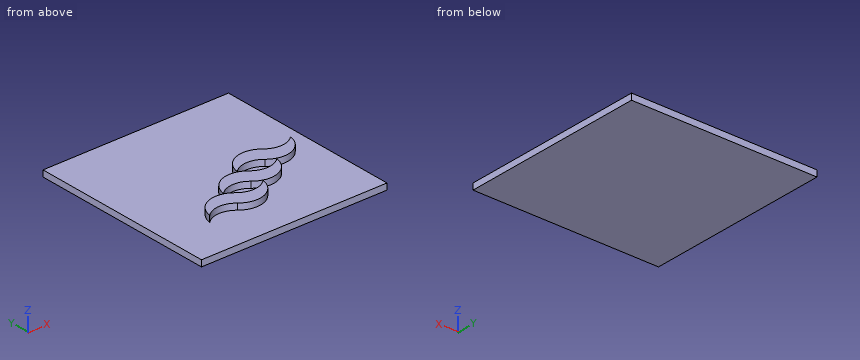
```python
from build123d import *

# Parameters (mm, degrees)
SKICA1_W                = 300
SKICA1_H                = 300
P_IDAT_VYSUNUT_M1_DEPTH = 10
P_IDAT_VYSUNUT_M3_DEPTH = 10


with BuildPart() as part:
    # Skica1 → Přidat vysunutím1 (new body)
    with BuildSketch(Plane.XY):
        with Locations((150, 150)):
            Rectangle(SKICA1_W, SKICA1_H)
    extrude(amount=P_IDAT_VYSUNUT_M1_DEPTH)

    # Skica3 → Přidat vysunutím3 (add)
    with BuildSketch(Plane.XY.offset(10)):
        with BuildLine():
            ThreePointArc((115.351436594, 67.036617417), (152.787337691, 60.386270146), (176.568555926, 90.053212507))
            ThreePointArc((176.568555926, 90.053212507), (153.853792867, 80.346404756), (130.562326016, 88.573807107))
            ThreePointArc((130.562326016, 88.573807107), (93.126424919, 95.224154378), (69.345206683, 65.557212017))
            ThreePointArc((69.345206683, 65.557212017), (92.059969742, 75.264019769), (115.351436594, 67.036617417))
        make_face()
        with BuildLine():
            ThreePointArc((179.434133768, 119.807545389), (141.998232671, 126.45789266), (118.217014435, 96.790950299))
            ThreePointArc((118.217014435, 96.790950299), (140.931777494, 106.49775805), (164.223244346, 98.270355699))
            ThreePointArc((164.223244346, 98.270355699), (201.659145443, 91.620008428), (225.440363678, 121.286950789))
            ThreePointArc((225.440363678, 121.286950789), (202.725600619, 111.580143037), (179.434133768, 119.807545389))
        make_face()
        with BuildLine():
            ThreePointArc((228.30594152, 151.04128367), (190.870040423, 157.691630941), (167.088822187, 128.024688581))
            ThreePointArc((167.088822187, 128.024688581), (189.803585246, 137.731496332), (213.095052098, 129.504093981))
            ThreePointArc((213.095052098, 129.504093981), (250.530953195, 122.85374671), (274.31217143, 152.52068907))
            ThreePointArc((274.31217143, 152.52068907), (251.597408371, 142.813881319), (228.30594152, 151.04128367))
        make_face()
    extrude(amount=P_IDAT_VYSUNUT_M3_DEPTH)


solid = part.part
```
Source: CAD feature listing. Evaluate the final solid. Frame: model axes, mm. Give positions to 0.01 mm unless a question says otherwise; leave off trailing zeros. Write each loop counter-clockwise with the first axis right and the second up, starting at its lowest first coordinate (ties: lowest second). Pieces come first, ordered by that corner, then holes. Notation, with made-up numbers: (74, 56) - (118, 56) arc R37 ccw to (118, 92) - close; hole circle Ø4 at (72.5, 17). An arc over 180 degrees is marked (long way). One line per item, written item: value. Start each with the question number.
Q1. Section query C-C, the plane y = 260. Return the cut outline in (x, z).
Q2. Section query A-A, the plane z = 16.5. Return the cut outline in (x, y).
Q3. Section query B-B, the plane x = 209. Return the cut outline in (y, z), then the cut area to 3 significant figures.
Q4. First-contact query: pin 1 Ø1.5 at (y, z) = (74.5, 17.5) entering from -X; pin 2 Ø5 at (x, z) = (98, 17) entering from +Y; pin 3 Ø8 at (x, z) = (110.5, 17.5) entering from -Y. Flat tips, straight axial feed; report the tip coordinate or a pass-through.
Q5. Material intervals for probe 1 along Z at (x, y) = (176, 155.5); probe 2 along Y at (x, z) = (204, 18); probe 3 along Y at (x, z) = (213, 17), sorted ascending. Write a range as from..to.
Q6. Section query D-D, the plane x = 270.5. Return the cut outline in (y, z).
Answer:
1. outline: (0, 0) - (300, 0) - (300, 10) - (0, 10) - close
2. outline: (69.35, 65.56) arc R34.01 cw to (115.35, 67.04) arc R37.26 ccw to (176.57, 90.05) arc R34.01 cw to (130.56, 88.57) arc R37.26 ccw to start; (118.22, 96.79) arc R34.01 cw to (164.22, 98.27) arc R37.26 ccw to (225.44, 121.29) arc R34.01 cw to (179.43, 119.81) arc R37.26 ccw to start; (167.09, 128.02) arc R34.01 cw to (213.1, 129.5) arc R37.26 ccw to (274.31, 152.52) arc R34.01 cw to (228.31, 151.04) arc R37.26 ccw to start
3. outline: (0, 0) - (300, 0) - (300, 10) - (159.74, 10) - (159.74, 20) - (132.53, 20) - (132.53, 10) - (112.37, 10) - (112.37, 20) - (95.35, 20) - (95.35, 10) - (0, 10) - close
3. area: 3,440 mm2
4. pin 1: stops at x = 71.47
4. pin 2: stops at y = 97.16
4. pin 3: stops at y = 67.75
5. probe 1: z = 0..10
5. probe 2: y = 92.59..111.65, 135.12..160.08
5. probe 3: y = 98.38..113.52, 129.59..158.97
6. outline: (0, 0) - (300, 0) - (300, 10) - (149.3, 10) - (149.3, 20) - (140.59, 20) - (140.59, 10) - (0, 10) - close
